Autodesk Fusion 360 part; units mm, degrees
sketch "Sketch1" plane through (0, 0, 0) normal (0, 0, 1) x (1, 0, 0)
  circle A0 centre (0, 0) radius 12.5
  circle A1 centre (0, 0) radius 4
  dimension "d1" = 25
  dimension "d2" = 8
extrude "Extrude1" add sketch "Sketch1" along normal blind 7.6
sketch "Sketch2" plane through (0, 0, 7.6) normal (0, 0, 1) x (-1, 0, 0)
  circle A0 centre (0, 0) radius 4
  circle A1 centre (0, 0) radius 12.5
  circle A2 centre (0, 0) radius 18.85
  circle A3 centre (0, 0) radius 21.8
  dimension "d5" = 37.7
  dimension "d11" = 43.6
extrude "Extrude2" add sketch "Sketch2" along normal blind 7 contours A1 | A2
sketch "Sketch3" plane through (0, 0, 14.6) normal (0, 0, 1) x (-1, 0, 0)
  circle A0 centre (0, 0) radius 4
  circle A1 centre (0, 0) radius 18.85
  circle A2 centre (0, 0) radius 21.8
  dimension "d8" = 43.6
extrude "Extrude3" add sketch "Sketch3" along normal blind 1.5 contours A1 | A2
extrude "Extrude4" add sketch "Sketch2" against normal blind 1.5 contours A2 | A3
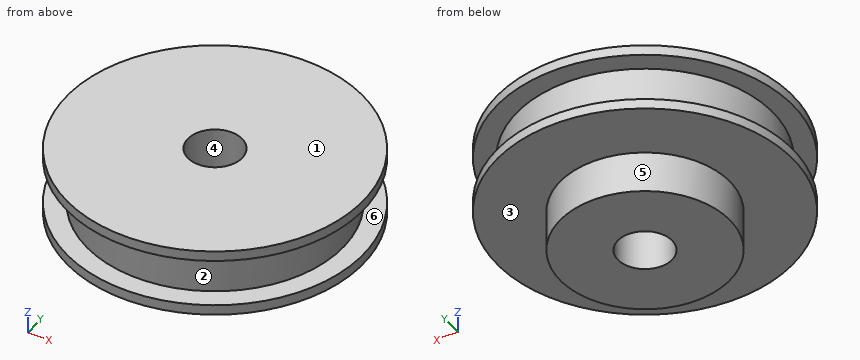
The listing builds one solid part. Answer for the finished solid, in the listing's coordinates (mm). Face numbers are marked on the shaded views. A direction names the side the tool comes from. Round coordinates to 2 decimals unless told otherwise and drop trailing zeros. Write each loop counter-clockwise with the first axis right and the second up, starting at its lowest first coordinate (ties: lowest second). Pieces come first, ordered by that corner, then holes. Notation, with made-up numbers: M 64,85 L 91,85 A12 cw 91,101 Z; hole C 66.25,61.5 d8. An arc over 180 degrees is marked long. Write each question's results on one line, items separated by ' | '. Start each with the question number.
Item 1: A cutting plane is placed at C-C on y = 17.5. Write down the section's boundary in (x, z).
Item 2: For the marked faces 1, 2 and 3, determine the directions among +Z, -Z, +X, -X, +Y, -Y from which every point of the face is accessible in a straight line to the end or side of a thin tool.
Item 3: A cutting plane is placed at D-D on x = -10. Write down the section's boundary in (y, z), and give its area (3 significant figures).
Item 4: Straight lines are drawn through the part: L1, parallel to X at y = 0, z = 11; L2, parallel to Z at x = -17.5, y = 8. For each, find the intervals that lie inside material, in ascending order. Write a range as [from, to].
Item 5: Flat-ended cylindrical pins translate along their axes: pin 1 Ø8 at (x, z) = (-5.5, 8.5) entering from -Y; pin 2 Ø8 at (x, z) = (3.5, 4.5) entering from +Y. Find the tip coordinate at first contact, or state that the pin passes through.
Item 6: For a pull along X with two mould halves and no side action, classify the marked faces 4, 5 and 6 as pulls with the +X half, pulls with the -X half, needs draft (parallel to the pull), parting line crosses it, or undercut.
Item 7: A cutting plane is placed at B-B on z = 3. Write down the section's boundary in (x, y).
Check sheet entries:
1) outline: M -13,6.1 L 13,6.1 L 13,7.6 L 7.01,7.6 L 7.01,14.6 L 13,14.6 L 13,16.1 L -13,16.1 L -13,14.6 L -7.01,14.6 L -7.01,7.6 L -13,7.6 Z
2) face 1: +Z, +X, -X, +Y, -Y | face 2: none | face 3: -Z
3) outline: M -19.37,6.1 L -7.5,6.1 L -7.5,0 L 7.5,0 L 7.5,6.1 L 19.37,6.1 L 19.37,7.6 L 15.98,7.6 L 15.98,14.6 L 19.37,14.6 L 19.37,16.1 L -19.37,16.1 L -19.37,14.6 L -15.98,14.6 L -15.98,7.6 L -19.37,7.6 Z | area: 431 mm²
4) L1: [-18.85, -4], [4, 18.85] | L2: [6.1, 7.6], [14.6, 16.1]
5) pin 1: y = -21.74 | pin 2: y = 21.8
6) face 4: undercut | face 5: parting line crosses it | face 6: needs draft
7) outline: C 0,0 d25; hole C 0,0 d8
